Input: part model. Units: mm. Frame: model coordinates. Give positions to 0.01 mm unless a question says otherwise; leave off trailing zeros. Loops run counter-clockwise (first coordinate to the right, second up) from the corner with the lowest first, then second, coordinate; pieces in that order, holes last. Notation, with made-up numbers: M 66,-4.5 L 71,-4.5 A21 ccw 71,21.5 Z; hole C 54,-6.75 d4. An arc over 180 degrees is marked long. Answer as a JSON object with one key per item and string values. Group by question number.
1) First-contact query: P1, Ø3, axis at x = 32.5, y = 7, coming from the +Z side; P2, Ø2, axis at y = 2.5, z = -2, coming from the +X side. Flat tips, straight axial feed; report the tip coordinate or a pass-through.
2) Ray query, L1, parallel to X at y = 7.75, z = 0.5; L2, parallel to Y at x = 42.5, z = 2.75; L3, parallel to Y at x = 44.5, z = -0.75. Return the intervals inside material, ascending.
3) Section query A-A on y = 7. Return loops of the section in (x, z), plus the area to 3 significant figures.
4) Section query B-B on x = 40.5. Return loops of the section in (y, z), plus the area to 3 significant figures.
5) Section query C-C on z = -1.5. Return loops of the section in (x, y).
from build123d import *

# Parameters (mm, degrees)
SKETCH1_R           = 50
SKETCH1_R_2         = 22.5
BOSS_EXTRUDE6_DEPTH = 10
SKETCH2_R           = 3.5
BOSS_EXTRUDE7_DEPTH = 100


with BuildPart() as part:
    # Sketch1 → Boss-Extrude6 (new body)
    with BuildSketch(Plane(origin=(0, 0, 0), x_dir=(1, 0, 0), z_dir=(0, 1, 0))):
        with Locations(Location((0, 0, 0), (0, 0, 270))):
            Circle(SKETCH1_R)
        with Locations(Location((0, 0, 0), (0, 0, 270))):
            Circle(SKETCH1_R_2, mode=Mode.SUBTRACT)
    extrude(amount=BOSS_EXTRUDE6_DEPTH)


with BuildPart() as body_2:
    # Sketch2 → Boss-Extrude7 (new body)
    with BuildSketch(Plane(origin=(10, 0, 0), x_dir=(0, 0, -1), z_dir=(1, 0, 0))):
        with Locations((0, 4.904618841)):
            Circle(SKETCH2_R)
    extrude(amount=BOSS_EXTRUDE7_DEPTH)


with BuildPart() as part_1:
    add(part.part)

    # Combine1: intersect body 2
    add(body_2.part, mode=Mode.INTERSECT)


solid = part_1.part
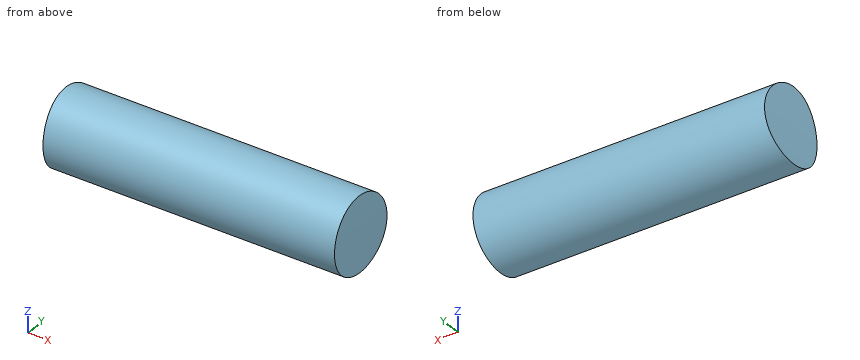
Output:
{
 "1": {"P1": "stops at z = 3.45", "P2": "stops at x = 49.99"},
 "2": {"L1": "x = 22.49 to 50", "L2": "y = 2.74 to 7.07", "L3": "y = 1.49 to 8.32"},
 "3": {"outline": "M 22.32,-2.8 L 49.92,-2.8 A50 ccw 49.92,2.8 L 22.32,2.8 A22.5 cw Z", "area": "154 mm^2"},
 "4": {"outline": "C 4.9,0 d7", "area": "38.5 mm^2"},
 "5": {"outline": "M 22.45,1.74 L 49.98,1.74 L 49.98,8.07 L 22.45,8.07 Z"}
}
